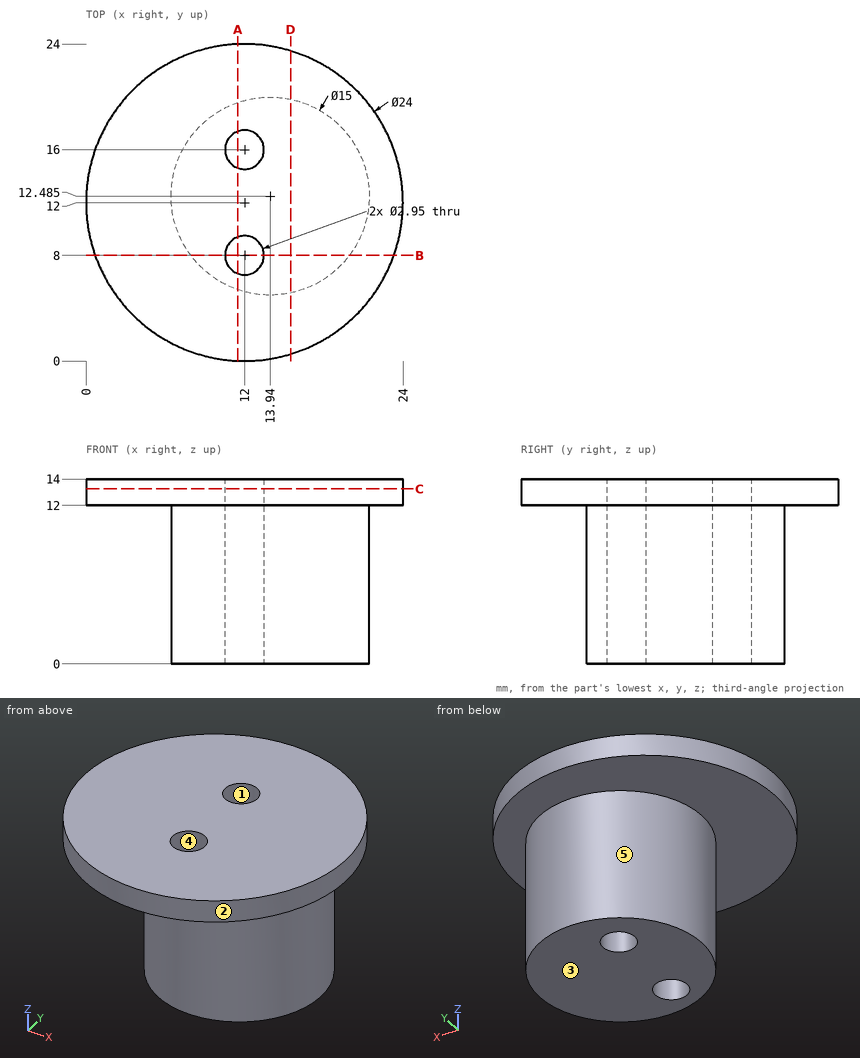
Answer from the drawing. Dimensions are ordinates in mm from the lowest x, y and z of the part. A direction names the side the tool comes from. Round coordinates to 2 decimals unless told otherwise and drop trailing zeros. Order: outer loops, then holes, each group sorted by start corner. A loop starts at its lowest first (then second) coordinate and runs counter-clockwise, first axis right, second up.
1) Flat-ended cylindrical pins translate along their axes: pin 1 (4 mm diameter, centred on x = 12, y = 16, fed in from -Z); pin 2 (2 mm diameter, centred on x = 18.5, z = 12.5, fed in from +Y) (1 decimal); pin 3 (1 mm diameter, centred on x = 18, z = 5.5, fed in from +Y); pin 4 (1.5 mm diameter, centred on x = 9.5, z = 10.5, fed in from -Y) (1 decimal). Find the tip coordinate at first contact, or state that the pin passes through.
2) The part is cut by section A-A on x = 11.5. Write down the section's boundary in (y, z).
3) The part is cut by section C-C on z = 13.25. Give the number of separate pieces and of enclosed holes in the cut face, plus the area to 3 significant figures.
4) The mould has two halves that part along Y. Classify the marked faces 1, 2 and 3: released by +Y, released by -Y, zero draft, split by the parting line, or undercut.
5) For the marked faces 4 and 5, determine the directions among +Z, -Z, +X, -X, +Y, -Y from which every point of the face is accessible in a straight line to the end or side of a thin tool.
6) The part is cut by section B-B on y = 8. Write down the section's boundary in (x, z) (1 decimal), plus the area to 3 significant figures.
7) The part is cut by section D-D on x = 15.5. Write down the section's boundary in (y, z), plus the area to 3 significant figures.
8) Straight lines are drawn through the part: L1, parallel to Y at x = 12, z = 5.5 (1 decimal); L2, parallel to Z at x = 5.5, y = 12.5; L3, parallel to X at y = 9.25, z = 11 (1 decimal). For each, find the intervals that lie inside material, in ascending order.
Resolved:
1. pin 1: stops at z = 0
1. pin 2: stops at y = 22.7
1. pin 3: stops at y = 19.09
1. pin 4: stops at y = 6
2. outline: (0.01, 12) - (5.39, 12) - (5.39, 0) - (6.61, 0) - (6.61, 14) - (0.01, 14) - close; (9.39, 0) - (14.61, 0) - (14.61, 14) - (9.39, 14) - close; (17.39, 0) - (19.58, 0) - (19.58, 12) - (23.99, 12) - (23.99, 14) - (17.39, 14) - close
3. separate pieces: 1
3. enclosed holes: 2
3. area: 439 mm2
4. face 1: undercut
4. face 2: split by the parting line
4. face 3: zero draft
5. face 4: +Z, -Z
5. face 5: -Z
6. outline: (0.7, 12) - (7.9, 12) - (7.9, 0) - (10.5, 0) - (10.5, 14) - (0.7, 14) - close; (13.5, 0) - (20, 0) - (20, 12) - (23.3, 12) - (23.3, 14) - (13.5, 14) - close
6. area: 148 mm2
7. outline: (0.52, 12) - (5.15, 12) - (5.15, 0) - (19.82, 0) - (19.82, 12) - (23.48, 12) - (23.48, 14) - (0.52, 14) - close
7. area: 222 mm2
8. L1: y = 5.2 to 6.5, 9.5 to 14.5, 17.5 to 19.7
8. L2: z = 12 to 14
8. L3: x = 7.2 to 11.2, 12.8 to 20.7
